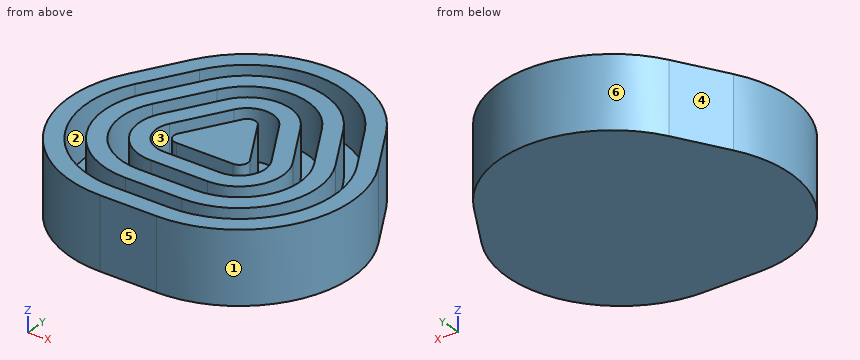
```python
from build123d import *

# Parameters (mm, degrees)
F1_DEPTH = 57
F3_DEPTH = 25


with BuildPart() as f1:
    # F0 (on Top) → F1 (new body)
    with BuildSketch(Plane.XY):
        with BuildLine():
            ThreePointArc((8.6602540378, 32.4022103819), (0, 37.4022103819), (-8.6602540378, 32.4022103819))
            Line((-8.6602540378, 32.4022103819), (-41.3397459622, -24.2003299966))
            ThreePointArc((-41.3397459622, -24.2003299966), (-41.3397459622, -34.2003299966), (-32.6794919243, -39.2003299966))
            Line((-32.6794919243, -39.2003299966), (32.6794919243, -39.2003299966))
            ThreePointArc((32.6794919243, -39.2003299966), (41.3397459622, -34.2003299966), (41.3397459622, -24.2003299966))
            Line((41.3397459622, -24.2003299966), (8.6602540378, 32.4022103819))
        make_face()
    extrude(amount=F1_DEPTH)



with BuildPart() as f1b:
    # F0 (on Top) → F1, piece 2 (new body)
    with BuildSketch(Plane.XY):
        with BuildLine():
            Line((75.9807621135, -4.2003299966), (43.3012701892, 52.4022103819))
            ThreePointArc((43.3012701892, 52.4022103819), (0, 77.4022103819), (-43.3012701892, 52.4022103819))
            Line((-43.3012701892, 52.4022103819), (-75.9807621135, -4.2003299966))
            ThreePointArc((-75.9807621135, -4.2003299966), (-75.9807621135, -54.2003299966), (-32.6794919243, -79.2003299966))
            Line((-32.6794919243, -79.2003299966), (32.6794919243, -79.2003299966))
            ThreePointArc((32.6794919243, -79.2003299966), (75.9807621135, -54.2003299966), (75.9807621135, -4.2003299966))
        make_face()
        with BuildLine():
            ThreePointArc((-25.9807621135, 42.4022103819), (0, 57.4022103819), (25.9807621135, 42.4022103819))
            Line((25.9807621135, 42.4022103819), (58.6602540378, -14.2003299966))
            ThreePointArc((58.6602540378, -14.2003299966), (58.6602540378, -44.2003299966), (32.6794919243, -59.2003299966))
            Line((32.6794919243, -59.2003299966), (-32.6794919243, -59.2003299966))
            ThreePointArc((-32.6794919243, -59.2003299966), (-58.6602540378, -44.2003299966), (-58.6602540378, -14.2003299966))
            Line((-58.6602540378, -14.2003299966), (-25.9807621135, 42.4022103819))
        make_face(mode=Mode.SUBTRACT)
    extrude(amount=F1_DEPTH)


with BuildPart() as f1c:
    # F0 (on Top) → F1, piece 3 (new body)
    with BuildSketch(Plane.XY):
        with BuildLine():
            Line((110.6217782649, 15.7996700034), (77.9422863406, 72.4022103819))
            ThreePointArc((77.9422863406, 72.4022103819), (0, 117.4022103819), (-77.9422863406, 72.4022103819))
            Line((-77.9422863406, 72.4022103819), (-110.6217782649, 15.7996700034))
            ThreePointArc((-110.6217782649, 15.7996700034), (-110.6217782649, -74.2003299966), (-32.6794919243, -119.2003299966))
            Line((-32.6794919243, -119.2003299966), (32.6794919243, -119.2003299966))
            ThreePointArc((32.6794919243, -119.2003299966), (110.6217782649, -74.2003299966), (110.6217782649, 15.7996700034))
        make_face()
        with BuildLine():
            ThreePointArc((-60.6217782649, 62.4022103819), (0, 97.4022103819), (60.6217782649, 62.4022103819))
            Line((60.6217782649, 62.4022103819), (93.3012701892, 5.7996700034))
            ThreePointArc((93.3012701892, 5.7996700034), (93.3012701892, -64.2003299966), (32.6794919243, -99.2003299966))
            Line((32.6794919243, -99.2003299966), (-32.6794919243, -99.2003299966))
            ThreePointArc((-32.6794919243, -99.2003299966), (-93.3012701892, -64.2003299966), (-93.3012701892, 5.7996700034))
            Line((-93.3012701892, 5.7996700034), (-60.6217782649, 62.4022103819))
        make_face(mode=Mode.SUBTRACT)
    extrude(amount=F1_DEPTH)


with BuildPart() as f1d:
    # F0 (on Top) → F1, piece 4 (new body)
    with BuildSketch(Plane.XY):
        with BuildLine():
            Line((145.2627944163, 35.7996700034), (112.583302492, 92.4022103819))
            ThreePointArc((112.583302492, 92.4022103819), (0, 157.4022103819), (-112.583302492, 92.4022103819))
            Line((-112.583302492, 92.4022103819), (-145.2627944163, 35.7996700034))
            ThreePointArc((-145.2627944163, 35.7996700034), (-145.2627944163, -94.2003299966), (-32.6794919243, -159.2003299966))
            Line((-32.6794919243, -159.2003299966), (32.6794919243, -159.2003299966))
            ThreePointArc((32.6794919243, -159.2003299966), (145.2627944163, -94.2003299966), (145.2627944163, 35.7996700034))
        make_face()
        with BuildLine():
            ThreePointArc((-95.2627944163, 82.4022103819), (0, 137.4022103819), (95.2627944163, 82.4022103819))
            Line((95.2627944163, 82.4022103819), (127.9422863406, 25.7996700034))
            ThreePointArc((127.9422863406, 25.7996700034), (127.9422863406, -84.2003299966), (32.6794919243, -139.2003299966))
            Line((32.6794919243, -139.2003299966), (-32.6794919243, -139.2003299966))
            ThreePointArc((-32.6794919243, -139.2003299966), (-127.9422863406, -84.2003299966), (-127.9422863406, 25.7996700034))
            Line((-127.9422863406, 25.7996700034), (-95.2627944163, 82.4022103819))
        make_face(mode=Mode.SUBTRACT)
    extrude(amount=F1_DEPTH)


with BuildPart() as f1_1:
    add(f1.part)

    add(f1b.part)  # F3 merges F1b

    add(f1c.part)  # F3 merges F1c

    add(f1d.part)  # F3 merges F1d
    # F2 (on face) → F3 (join)
    with BuildSketch(Plane(origin=(0, 0, 0), x_dir=(1, 0, 0), z_dir=(0, 0, -1))):
        with BuildLine():
            ThreePointArc((-32.6794919243, 159.2003299966), (-145.2627944163, 94.2003299966), (-145.2627944163, -35.7996700034))
            Line((-145.2627944163, -35.7996700034), (-112.583302492, -92.4022103819))
            ThreePointArc((-112.583302492, -92.4022103819), (0, -157.4022103819), (112.583302492, -92.4022103819))
            Line((112.583302492, -92.4022103819), (145.2627944163, -35.7996700034))
            ThreePointArc((145.2627944163, -35.7996700034), (145.2627944163, 94.2003299966), (32.6794919243, 159.2003299966))
            Line((32.6794919243, 159.2003299966), (-32.6794919243, 159.2003299966))
        make_face()
    extrude(amount=F3_DEPTH)


solid = f1_1.part
```
Here's how the part is built. I have some questions about the finished solid (model axes, mm). Face numbers are marked on the shaded views. A direction names the side the tool comes from. Coordinates: 2 decimals unless noted, no trailing zeros. Loops run counter-clockwise (first coordinate to the right, second up) from the corner with the lowest first, then second, coordinate; pieces in that order, holes last. Notation, with made-up numbers: M 36,1 L 50,1 A33 cw 50,30 Z; hole C 58,33.5 d3. An arc over 180 degrees is marked long. One line per item, written item: value.
1. Please list where these lines run through material, in increasing order: probe 1 along Y at (x, z) = (-68.5, 20); probe 2 along X at (y, z) = (-89, 49) (3 decimals); probe 3 along Y at (x, z) = (-48, 22).
Geometry says:
probe 1: y = -154.17 to -133.2, -111.76 to -89.34, -64.08 to 8.76, 48.76 to 85.78, 113.47 to 137.89
probe 2: x = -148.109 to -125.005, -99.94 to -69.066, 69.066 to 99.94, 125.005 to 148.109
probe 3: y = -158.29 to -138.13, -117.89 to -97.5, -76.8 to -54.99, 4.26 to 44.26, 78.35 to 103.53, 126.38 to 148.22
2. Imagine slicing it at D-D (y = 113.5). List the corners of the cut face in (x, z) for me.
Geometry says:
outline: M -97.4,-25 L 97.4,-25 L 97.4,57 L 68.46,57 L 68.46,0 L 26.21,0 L 26.21,57 L -26.21,57 L -26.21,0 L -68.46,0 L -68.46,57 L -97.4,57 Z
3. Will these pins go through, and if not, where does the flat tip stop? pin 1 Ø2 at (x, z) = (-36.5, -6) entering from -Y; pin 2 Ø1.5 at (x, y) = (-64, 21) entering from +Z; pin 3 Ø1 at (x, z) = (-58.5, 36.5) entering from -Y.
Geometry says:
pin 1: stops at y = -159.17
pin 2: stops at z = 0
pin 3: stops at y = -156.71
4. Imagine slicing it at C-C (x = -47). List the corners of the cut face in (y, z) for me.
Geometry says:
outline: M -158.41,-25 L 148.61,-25 L 148.61,57 L 126.86,57 L 126.86,0 L 104.16,0 L 104.16,57 L 79.28,57 L 79.28,0 L 46,0 L 46,57 L 6,57 L 6,0 L -55.56,0 L -55.56,57 L -77.11,57 L -77.11,0 L -97.72,0 L -97.72,57 L -118.05,57 L -118.05,0 L -138.26,0 L -138.26,57 L -158.41,57 Z
5. Imagine slicing it at A-A (z = 37.5). State how many separate pieces and enclosed holes the cut face has, and give its area (3 significant figures).
Geometry says:
separate pieces: 4
enclosed holes: 3
area: 46,000 mm2
6. Thinking about a two-plate mould opening in X: for the marked faces 3, 4, 5 and 6, which applies, +X half, -X half, draft (parallel to the pull), parting line (faces both ways), or undercut?
Geometry says:
face 3: undercut
face 4: -X half
face 5: draft
face 6: parting line
7. Imagine slicing it at B-B (y = -68). List the corners of the cut face in (x, z) for me, and give its area (3 significant figures).
Geometry says:
outline: M -156.75,-25 L 156.75,-25 L 156.75,57 L 135.61,57 L 135.61,0 L 113.89,0 L 113.89,57 L 90.94,57 L 90.94,0 L 64.22,0 L 64.22,57 L -64.22,57 L -64.22,0 L -90.94,0 L -90.94,57 L -113.89,57 L -113.89,0 L -135.61,0 L -135.61,57 L -156.75,57 Z
area: 20,200 mm2
8. On a 3-axis mill with a long thin cutter (end or side, diameter ignored), from which of +Z, -Z, +X, -X, +Y, -Y can I reach the whole of each face in a straight line? I mean the marked faces 1 and 2. Say none if no direction works.
Geometry says:
face 1: +Z, -Z, +X
face 2: +Z
